Geometry check sheet. Reference: drawing and pictorial views, mm from the part's lowest x, y, z. A direction names the side the tool comes from. Give positions to 0.01 mm unless a question says otherwise; leave off trailing zeros. Loops run counter-clockwise (first coordinate to the right, second up) from the corner with the lowest first, then second, coordinate; pieces in that order, holes last. Notation, with made-up numbers: (46, 17.5) - (100, 17.5) arc R15 cw to (100, 39.5) - close; hole circle Ø7 at (28.25, 29.25). An arc over 180 degrees is marked (long way). Use CSV: the item, a comma, the result in double quotes.
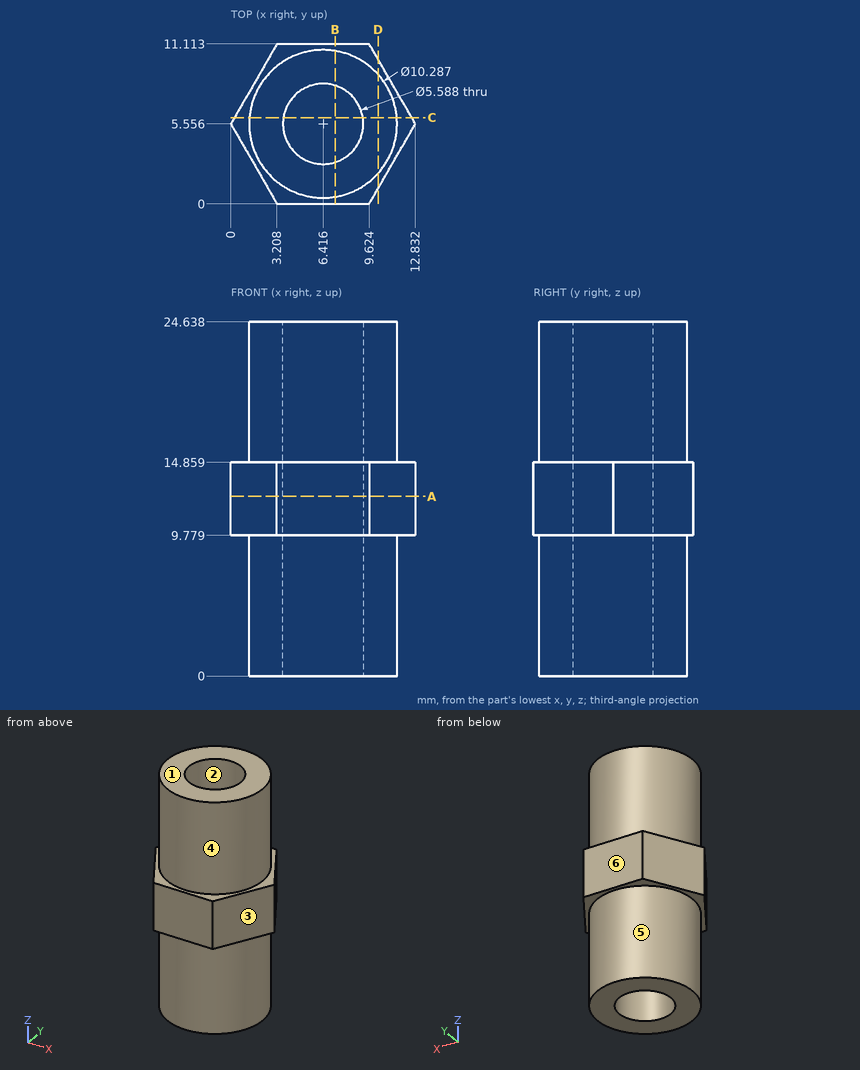
1. Release check for a two-part mould opening along X. For the marked faces 1, 2 and 3 record: released by +X, released by -X, zero draft, split by the parting line, or undercut.
Completed:
face 1,"zero draft"
face 2,"undercut"
face 3,"released by +X"
2. Scan lines: line 1 along X through (y, z) = (5.5, 6.5); line 2 along X through (y, z) = (4.5, 9); line 3 along Y through (x, z) = (8.75, 20) (1 decimal). Record each from-to range of solid material in increasing order.
Completed:
line 1,"x = 1.27 to 3.62, 9.21 to 11.56"
line 2,"x = 1.38 to 3.83, 9 to 11.45"
line 3,"y = 1 to 4, 7.1 to 10.1"
3. Sectioned sample at A-A, the plane z = 12.5. Record the boundary of the cut face in (x, y) (1 decimal).
Completed:
outline,"(0, 5.6) - (3.2, 0) - (9.6, 0) - (12.8, 5.6) - (9.6, 11.1) - (3.2, 11.1) - close; hole circle Ø5.6 at (6.4, 5.6)"
4. Go/stop test with flat-tipped pins: pin 1 Ø1 at (y, z) = (9.5, 15.5) entering from +X (1 decimal); pin 2 Ø5.5 at (x, y) = (5.5, 5) entering from +Z; pin 3 Ø6 at (x, z) = (6, 19.5) entering from +Y; pin 4 Ø1 at (y, z) = (7, 4.5) entering from -X. Record where each tip stops, or that it passes through.
Completed:
pin 1,"stops at x = 10.2"
pin 2,"stops at z = 24.64"
pin 3,"stops at y = 10.7"
pin 4,"stops at x = 1.36"
5. Sectioned sample at C-C, the plane y = 6. Record the boundary of the cut face in (x, z) (1 decimal).
Completed:
outline,"(0.3, 9.8) - (1.3, 9.8) - (1.3, 0) - (3.7, 0) - (3.7, 24.6) - (1.3, 24.6) - (1.3, 14.9) - (0.3, 14.9) - close; (9.2, 0) - (11.5, 0) - (11.5, 9.8) - (12.6, 9.8) - (12.6, 14.9) - (11.5, 14.9) - (11.5, 24.6) - (9.2, 24.6) - close"
6. Sectioned sample at D-D, the plane x = 10.25. Record the boundary of the cut face in (y, z) (1 decimal).
Completed:
outline,"(1.1, 9.8) - (2.1, 9.8) - (2.1, 0) - (9, 0) - (9, 9.8) - (10, 9.8) - (10, 14.9) - (9, 14.9) - (9, 24.6) - (2.1, 24.6) - (2.1, 14.9) - (1.1, 14.9) - close"
7. Set-up check for the marked faces 4, 5 and 6: record each of +Z, -Z, +X, -X, +Y, -Y from which the full face is reachable in a straight line by a thin tool's end or side.
Completed:
face 4,"+Z"
face 5,"-Z"
face 6,"+Z, -Z, +X, -X, +Y"
8. Sectioned sample at B-B, the plane x = 7.25. Record the boundary of the cut face in (y, z).
Completed:
outline,"(0, 9.78) - (0.48, 9.78) - (0.48, 0) - (2.89, 0) - (2.89, 24.64) - (0.48, 24.64) - (0.48, 14.86) - (0, 14.86) - close; (8.22, 0) - (10.63, 0) - (10.63, 9.78) - (11.11, 9.78) - (11.11, 14.86) - (10.63, 14.86) - (10.63, 24.64) - (8.22, 24.64) - close"
